Autodesk Inventor part; units mm, degrees
ref_plane "Work Plane1" through (10, 22.9435, 44.4702) normal (1, 0, 0) x (0, 1, 0)
ref_plane "XZ Plane" through (0, 0, 0) normal (0, 1, 0) x (-1, 0, 0)
ref_plane "XY Plane" through (0, 0, 0) normal (0, 0, 1) x (1, 0, 0)
sketch "Sketch1" plane through (0, 0, 0) normal (1, 0, 0) x (0, 1, 0)
  line L0 (0, 0) -> (0, -180)
  line L1 (0, -180) -> (21.1309, -225.3154)
  line L2 (21.1309, -225.3154) -> (22.9435, -224.4702)
  line L3 (22.9435, -224.4702) -> (2.2068, -180)
  line L4 (2.2068, -180) -> (2.2068, 0)
  line L5 (2.2068, 0) -> (22.9435, 44.4702)
  line L6 (22.9435, 44.4702) -> (21.1309, 45.3154)
  line L7 (0, 0) -> (21.1309, 45.3154)
  line L8 (0, 0) -> (67.9565, 0) construction
  dimension "d0" = 180
  dimension "d1" = 25
  dimension "d2" = 25
  dimension "d3" = 2
  dimension "d4" = 50
  dimension "d5" = 50
extrude "base" add sketch "Sketch1" along normal blind 20
sketch "Sketch2" plane through (0, 2.2068, 0) normal (0, 1, 0) x (1, 0, 0)
  circle A0 centre (10, 10) radius 3
  circle A1 centre (10, 146.5) radius 3
  line L0 (0, 0) -> (20, 0) construction
  line L1 (10, 0) -> (10, 23.1136) construction
  dimension "d8" = 6
  dimension "d9" = 6
  dimension "d10" = 10
  dimension "d11" = 136.5
extrude "holes" cut sketch "Sketch2" against normal blind 25
sketch "Sketch3" plane through (0, 2.2068, -180) normal (0, 0.9063, 0.4226) x (1, 0, 0)
  line L0 (0, 49.0674) -> (20, 49.0674) construction
  line L1 (10, 49.0674) -> (10, 4.5106) construction
  point P0 (0, -164.068)
  point P1 (10, 19.0674)
  dimension "d14" = 30
hole "ballastHole_originalAtTheFront" [suppressed]
sketch "Sketch4" plane through (0, 2.2068, 0) normal (0, 1, 0) x (1, 0, 0)
  line L0 (0, 0) -> (20, 0)
  line L1 (0, 180) -> (20, 180)
  line L2 (10, 180) -> (10, 136)
  dimension "d30" = 44
hole "ballastHole" [suppressed]
sketch "Sketch5" plane through (0, 2.2068, -180) normal (0, 0.9063, 0.4226) x (1, 0, 0)
  line L0 (0, 0) -> (20, 0) construction
  line L1 (10, 0) -> (10, 49.0674) construction
  line L2 (0, 49.0674) -> (20, 49.0674) construction
  arc A0 (7, 9.5337) -> (13, 9.5337) centre (10, 9.5337) ccw
  line L3 (10, 9.5337) -> (7, 9.5337) construction
  line L4 (10, 9.5337) -> (13, 9.5337) construction
  line L5 (7, 9.5337) -> (7, 39.5337)
  line L6 (13, 9.5337) -> (13, 39.5337)
  arc A1 (13, 39.5337) -> (7, 39.5337) centre (10, 39.5337) ccw
  line L7 (10, 39.5337) -> (13, 39.5337) construction
  line L8 (10, 39.5337) -> (7, 39.5337) construction
  point P0 (0, -164.068)
  point P1 (10, 6.5337)
  dimension "d31" = 180
  dimension "d32" = 3
  dimension "d33" = 30
  dimension "d34" = 180
  dimension "d35" = 49.0674
  dimension "d36" = 6.5337
extrude "Extrusion3" cut sketch "Sketch5" against normal blind 10
sketch "Sketch6" plane through (0, 22.9435, 44.4702) normal (0, 0.9063, -0.4226) x (1, 0, 0)
  line L0 (0, 0) -> (20, 0) construction
  line L1 (10, 0) -> (10, 50) construction
  line L2 (0, 50) -> (20, 50) construction
  arc A0 (4, 12.0337) -> (16, 12.0337) centre (10, 12.0337) ccw
  line L3 (10, 12.0337) -> (16, 12.0337) construction
  line L4 (10, 12.0337) -> (4, 12.0337) construction
  line L5 (4, 12.0337) -> (4, 37.0337)
  line L6 (16, 12.0337) -> (16, 37.0337)
  line L7 (0, 49.0674) -> (20, 49.0674) construction
  arc A1 (16, 37.0337) -> (4, 37.0337) centre (10, 37.0337) ccw
  line L8 (10, 37.0337) -> (16, 37.0337) construction
  line L9 (10, 37.0337) -> (4, 37.0337) construction
  point P0 (10, 6.0337)
  dimension "d39" = 180
  dimension "d40" = 6
  dimension "d41" = 25
  dimension "d42" = 49.0674
  dimension "d43" = 6.0337
  dimension "d44" = 180
extrude "Extrusion4" cut sketch "Sketch6" against normal blind 10
sketch "Sketch7" plane through (0, 2.2068, 0) normal (0, 1, 0) x (1, 0, 0)
  line L0 (0, 0) -> (20, 0) construction
  line L1 (10, 0) -> (10, 180) construction
  line L2 (0, 180) -> (20, 180) construction
  arc A0 (4, 23) -> (16, 23) centre (10, 23) ccw
  line L3 (10, 23) -> (16, 23) construction
  line L4 (10, 23) -> (4, 23) construction
  line L5 (4, 23) -> (4, 48)
  line L6 (16, 23) -> (16, 48)
  circle A1 centre (10, 10) radius 3 construction
  line L7 (10, 13) -> (24.9558, 13) construction
  arc A2 (16, 48) -> (4, 48) centre (10, 48) ccw
  line L8 (10, 48) -> (4, 48) construction
  line L9 (10, 48) -> (16, 48) construction
  line L10 (10, 64.875) -> (4, 64.875) construction
  line L11 (10, 64.875) -> (16, 64.875) construction
  arc A3 (4, 64.875) -> (16, 64.875) centre (10, 64.875) ccw
  line L12 (4, 64.875) -> (4, 89.875)
  line L13 (16, 64.875) -> (16, 89.875)
  line L14 (10, 89.875) -> (4, 89.875) construction
  line L15 (10, 89.875) -> (16, 89.875) construction
  arc A4 (16, 89.875) -> (4, 89.875) centre (10, 89.875) ccw
  circle A5 centre (10, 146.5) radius 3 construction
  line L16 (10, 143.5) -> (28.9866, 143.5) construction
  line L17 (10, 106.75) -> (4, 106.75) construction
  line L18 (10, 106.75) -> (16, 106.75) construction
  arc A6 (4, 106.75) -> (16, 106.75) centre (10, 106.75) ccw
  line L19 (4, 106.75) -> (4, 131.75)
  line L20 (16, 106.75) -> (16, 131.75)
  line L21 (10, 131.75) -> (4, 131.75) construction
  line L22 (10, 131.75) -> (16, 131.75) construction
  arc A7 (16, 131.75) -> (4, 131.75) centre (10, 131.75) ccw
  point P0 (10, 17)
  point P1 (10, 58.875)
  point P2 (10, 100.75)
  point P3 (10, 7)
  dimension "d47" = 180
  dimension "d48" = 6
  dimension "d49" = 25
  dimension "d52" = 180
  dimension "d55" = 41.875
  dimension "d62" = 130.5
  dimension "d68" = 7
  dimension "d69" = 10
extrude "Extrusion5" cut sketch "Sketch7" against normal blind 10
ref_plane "Work Plane1" through (10, 22.9435, 44.4702) normal (1, 0, 0) x (0, 1, 0)
equation "\"d9\" = d8"
equation "\"d55\" = d49 + d51 + 2 * d48"
equation "\"d51\" = -1.5 * d48 - 0.75 * d49 + 0.25 * d62"
properties part number "sled" material "Steel"
Model file for the job. Use its own axes, mm. A direction names the side the tool comes from. Give positions to 0.01 mm unless a question says otherwise; leave off trailing zeros. Loops run counter-clockwise (first coordinate to the right, second up) from the corner with the lowest first, then second, coordinate; pieces in that order, holes last.
Item 1: Slice it at B-B (y = 10.75). Write the cut outline in (x, z).
Check values:
outline: (0, -203.05) - (7, -203.05) - (7, -198.32) - (0, -198.32) - close; (0, 18.32) - (4, 18.32) - (4, 23.05) - (0, 23.05) - close; (13, -203.05) - (20, -203.05) - (20, -198.32) - (13, -198.32) - close; (16, 18.32) - (20, 18.32) - (20, 23.05) - (16, 23.05) - close
Item 2: Which spindle directions (+Z, -Z, +X, -X, +Y, -Y) get a long thin tool onto all of the face, cutting with end or side? Do faces 1 (the face through (10, 1, -17)), 2 (the face through (9.868, 19.499, 39.417)), 3 (the face through (3.2, 10.4, 22.3)). Say none if no direction does.
Check values:
face 1: +Y, -Y
face 2: -Y
face 3: +Z, +X, -X, -Y
Item 3: Mould opens along X. For faces 4 (the face through (7, 12, -202)), 5 (the face through (10.13, 1.12, -137.75)), 6 (the face through (0, 2, -89)), 7 (the face through (5.4, 10.4, -202.3)) say: +X half, -X half, draft (parallel to the pull), parting line (faces both ways), or undercut.
Check values:
face 4: undercut
face 5: undercut
face 6: -X half
face 7: draft
Item 4: Drill centre lines: line 1 along X through (y, z) = (1.75, -146.5); line 2 along Z through (x, y) = (5.5, 1.75); line 3 along Z through (x, y) = (10, 1.7) (3 decimals). Where is each one in solid material? Low to high.
Check values:
line 1: x = 0 to 7, 13 to 20
line 2: z = -183.75 to -135.72, -102.78 to -93.84, -60.91 to -51.97, -19.03 to 3.75
line 3: z = -183.646 to -149.5, -143.5 to -137.75, -100.75 to -95.875, -58.875 to -54, -17 to -13, -7 to 3.646
Item 5: Drop flat-ended pins along their axis: P1, Ø2, axis at x = 6, y = 18, coming from the +Z side; P2, Ø6, axis at x = 13, z = -102.5, coming from the +Y side; P3, Ø5, axis at x = 7, y = 11.5, coming from the +Z side. Give the stop position or say it passes through.
Check values:
P1: stops at z = 40.75
P2: stops at y = 2.21
P3: stops at z = -194.57
Item 6: Slice it at A-A (z = -146.5). Write the cut outline in (x, y).
Check values:
outline: (0, 0) - (7, 0) - (7, 2.21) - (0, 2.21) - close; (13, 0) - (20, 0) - (20, 2.21) - (13, 2.21) - close
Item 7: Slice it at D-D (x = 10). Give the number of separate pieces and of enclosed holes in the cut face, plus the area to 3 significant figures.
Check values:
separate pieces: 8
enclosed holes: 0
area: 178 mm2
Item 8: Slice it at C-C (z = 28.5). Write the cut outline in (x, y).
Check values:
outline: (0, 13.29) - (4, 13.29) - (4, 15.5) - (0, 15.5) - close; (16, 13.29) - (20, 13.29) - (20, 15.5) - (16, 15.5) - close
